The model under review builds one solid part; all positions refer to its coordinate system, in mm. Coordinates: 2 decimals unless noted, no trailing zeros. Order: outer loops, then holes, each group sorted by start corner. A loop starts at its lowest first (then second) coordinate and runs counter-clockwise, first axis right, second up. Notation, with made-up numbers: (63, 4) -> (106, 4) arc R20 cw to (106, 11) -> close; hole circle Ø8 at (-2.75, 66). An arc over 180 degrees is marked (long way). Use one line per item in the form item = value. Start each with the question number.
(1) Take a section at C-C (z = 519). State the section outline as (x, y) points, then the cut area to 3 significant figures.
(2) Take a section at A-A (y = -4.5). State the section outline as (x, z) points.
(3) Insertion check: pin 1 Ø12 at (y, z) = (-5, 532.5) entering from -X; pin 2 Ø10 at (y, z) = (-13, 572.5) entering from -X; pin 3 Ø1 at (x, y) = (152, 10) entering from +Z. Each pin has a flat end and moves straight along its axis. Give the tip position at first contact, or say it passes through.
(4) Take a section at B-B (x = 441). State the section outline as (y, z) points.
(5) Wall thickness on line 1 along Z through (x, y) = (98.5, 11); line 2 along X through (y, z) = (-8.5, 288); line 3 along X through (y, z) = (10, 539.5): over which ranges is each line inside the solid? List them lowest first.
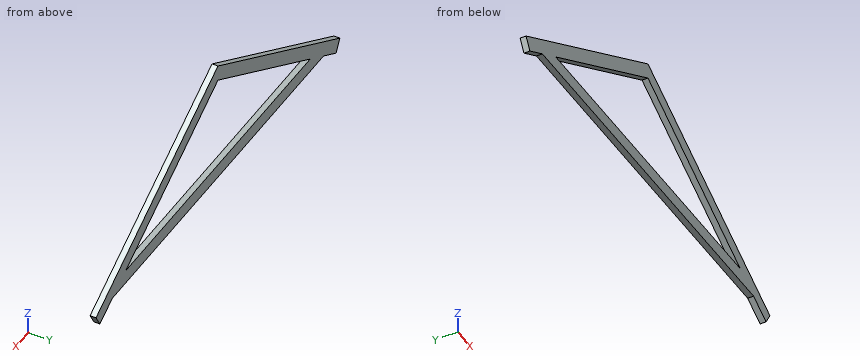
```python
from build123d import *

# Parameters (mm, degrees)
F1_DEPTH = 19.05


with BuildPart() as f1:
    # F0 (on Front) → F1 (new body, symmetric)
    with BuildSketch(Plane.XZ):
        Polygon((-1334.847673, -224.800255), (-1190.686777, -141.568923), (1247.713223, -141.568923), (1391.874119, -224.800255), (1436.324119, -147.810597), (28.513223, 664.989403), (-1379.297673, -147.810597), align=None)
        Polygon((1093.733906, -52.668923), (-1036.70746, -52.668923), (28.513223, 562.336525), align=None, mode=Mode.SUBTRACT)
    extrude(amount=F1_DEPTH, both=True)


solid = f1.part
```
Findings:
q1.outline = (-224.35, -19.05) -> (-46.55, -19.05) -> (-46.55, 19.05) -> (-224.35, 19.05) -> close; (103.57, -19.05) -> (281.37, -19.05) -> (281.37, 19.05) -> (103.57, 19.05) -> close
q1.area = 13,500 mm²
q2.outline = (-1379.3, -147.81) -> (-1334.85, -224.8) -> (-1190.69, -141.57) -> (1247.71, -141.57) -> (1391.87, -224.8) -> (1436.32, -147.81) -> (28.51, 664.99) -> close; hole (-1036.71, -52.67) -> (1093.73, -52.67) -> (28.51, 562.34) -> close
q3.pin_1 = -211.36
q3.pin_2 = -140.34
q3.pin_3 = 593.98
q4.outline = (-19.05, -141.57) -> (19.05, -141.57) -> (19.05, -52.67) -> (-19.05, -52.67) -> close; (-19.05, 324.19) -> (19.05, 324.19) -> (19.05, 426.84) -> (-19.05, 426.84) -> close
q5.line_1 = -141.57 to -52.67, 521.93 to 624.58
q5.line_2 = -624.45 to -446.65, 503.68 to 681.48
q5.line_3 = -188.84 to -11.04, 68.07 to 245.87
